from build123d import *

# Parameters (mm, degrees)
SKETCH1_W             = 24.5
SKETCH1_H             = 18.25
BOSS_EXTRUDE1_DEPTH   = 3
CHAMFER1_SIZE         = 0.75
CHAMFER2_SIZE         = 1.5
CHAMFER2_SIZE2        = 5.598076211
CHAMFER2_PART_2_SIZE  = 1.5
CHAMFER2_PART_2_SIZE2 = 5.598076211
CHAMFER2_PART_3_SIZE  = 1.5
CHAMFER2_PART_3_SIZE2 = 5.598076211
CHAMFER2_PART_4_SIZE  = 1.5
CHAMFER2_PART_4_SIZE2 = 5.598076211
SKETCH4_W             = 3
SKETCH4_H             = 0.5
BOSS_EXTRUDE2_DEPTH   = 2.5
FILLET2_R             = 1
FILLET2_OF_MIRROR2_R  = 1
SKETCH5_R             = 0.75
BOSS_EXTRUDE3_DEPTH   = 0.5
CUT_EXTRUDE2_REACH    = 23.288
SKETCH6_R             = 0.5


with BuildPart() as part:
    # Sketch1 → Boss-Extrude1 (new body)
    with BuildSketch(Plane(origin=(0, 0, 0), x_dir=(1, 0, 0), z_dir=(0, 1, 0))):
        Rectangle(SKETCH1_W, SKETCH1_H)
    extrude(amount=BOSS_EXTRUDE1_DEPTH)

    # Chamfer1
    chamfer1_edges = [part.edges().sort_by_distance(p)[0] for p in [
        (12.25, 1.5, 9.125),
        (-12.25, 1.5, 9.125),
        (-12.25, 1.5, -9.125),
        (12.25, 1.5, -9.125),
    ]]
    chamfer(chamfer1_edges, length=CHAMFER1_SIZE)

    # Chamfer2
    chamfer2_edges = [part.edges().sort_by_distance(p)[0] for p in [
        (12.25, 3, 0),
    ]]
    chamfer2_side = [part.faces().sort_by_distance(p)[0] for p in [
        (12.25, 1.5, 0),
    ]]
    chamfer(chamfer2_edges, length=CHAMFER2_SIZE, length2=CHAMFER2_SIZE2, reference=chamfer2_side[0])

    # Chamfer2 part 2
    chamfer2_part_2_edges = [part.edges().sort_by_distance(p)[0] for p in [
        (0, 3, 9.125),
    ]]
    chamfer2_part_2_side = [part.faces().sort_by_distance(p)[0] for p in [
        (0, 1.5, 9.125),
    ]]
    chamfer(chamfer2_part_2_edges, length=CHAMFER2_PART_2_SIZE, length2=CHAMFER2_PART_2_SIZE2, reference=chamfer2_part_2_side[0])

    # Chamfer2 part 3
    chamfer2_part_3_edges = [part.edges().sort_by_distance(p)[0] for p in [
        (-12.25, 3, 0),
    ]]
    chamfer2_part_3_side = [part.faces().sort_by_distance(p)[0] for p in [
        (-12.25, 1.5, 0),
    ]]
    chamfer(chamfer2_part_3_edges, length=CHAMFER2_PART_3_SIZE, length2=CHAMFER2_PART_3_SIZE2, reference=chamfer2_part_3_side[0])

    # Chamfer2 part 4
    chamfer2_part_4_edges = [part.edges().sort_by_distance(p)[0] for p in [
        (0, 3, -9.125),
    ]]
    chamfer2_part_4_side = [part.faces().sort_by_distance(p)[0] for p in [
        (0, 1.5, -9.125),
    ]]
    chamfer(chamfer2_part_4_edges, length=CHAMFER2_PART_4_SIZE, length2=CHAMFER2_PART_4_SIZE2, reference=chamfer2_part_4_side[0])

    # Sketch4 → Boss-Extrude2 (add)
    with BuildSketch(Plane.XZ):
        with Locations((0, 7.775)):
            Rectangle(SKETCH4_W, SKETCH4_H)
    boss_extrude2 = extrude(amount=BOSS_EXTRUDE2_DEPTH)

    # Fillet2
    fillet2_edges = [part.edges().sort_by_distance(p)[0] for p in [
        (-1.5, -2.5, 7.775),
        (1.5, -2.5, 7.775),
    ]]
    fillet(fillet2_edges, radius=FILLET2_R)

    # Mirror2: Boss-Extrude2 across plane
    add(boss_extrude2.mirror(Plane.XY))

    # Fillet2 of Mirror2
    fillet2_of_mirror2_edges = [part.edges().sort_by_distance(p)[0] for p in [
        (-1.5, -2.5, -7.775),
        (1.5, -2.5, -7.775),
    ]]
    fillet(fillet2_of_mirror2_edges, radius=FILLET2_OF_MIRROR2_R)

    # Sketch5 → Boss-Extrude3 (add)
    with BuildSketch(Plane(origin=(0, 0, -8.025), x_dir=(-1, 0, 0), z_dir=(0, 0, -1))):
        with Locations((0, -1.5)):
            Circle(SKETCH5_R)
    extrude(amount=BOSS_EXTRUDE3_DEPTH)

    # Sketch6 → Cut-Extrude2 (cut, up to next)
    with BuildSketch(Plane.XY.offset(8.025), mode=Mode.PRIVATE) as cut_extrude2_sk1:
        with Locations((0, -1.5)):
            Circle(SKETCH6_R)
    cut_extrude2_tool1 = extrude(cut_extrude2_sk1.sketch, amount=-CUT_EXTRUDE2_REACH, mode=Mode.PRIVATE) & part.part
    add(cut_extrude2_tool1.solids().sort_by_distance((0, -1.5, 8.025))[0], mode=Mode.SUBTRACT)


solid = part.part
Can you work these out from the model? Positions are in its coordinate system, mm. A direction names the side the tool comes from. Round coordinates to 2 decimals unless told otherwise and drop trailing zeros. Loops run counter-clockwise (first coordinate to the right, second up) from the corner with the lowest first, then second, coordinate; pieces in that order, holes last. Notation, with made-up numbers: (0.5, -18) - (39.5, -18) arc R20 cw to (39.5, 9) - close; hole circle Ø4 at (-37.75, 7). An arc over 180 degrees is marked (long way). Use CSV: the item, a comma, the result in double quotes. Start each with the question number.
1) We'd pull the mould along Y, two halves only. Please class faces 6 (the cylindrical face through (-1.215, -2.199, 7.778)), 7 (the flat face through (12.25, 1, 0)), 8 (the cylindrical face through (0.098, -0.756, -8.272)): released by +Y, released by -Y, zero draft, split by the parting line, or undercut.
2) If we section it at C-C on z = -4: Write out the boundary of the cut face in (x, y) (3 decimals).
3) Please list where these lines run through material, in increasing order: probe 1 along Z at (x, y) = (1, -0.05) (3 decimals); probe 2 along Y at (x, z) = (-4.5, -1); probe 3 along Y at (x, z) = (-10.5, -0.25). Write a range as [from, to].
4) If we section it at A-A on x = 0: Write out the boundary of the cut face in (y, z) (3 decimals).
5) If we section it at B-B on x = -4.75: Write out the boundary of the cut face in (y, z) (3 decimals), plus the area to 3 significant figures.
6) For faces 1 (the flat face through (10.034, 2.094, 0.123)), 2 (the flat face through (-0.35, -0.95, 8.025)), 3 (the flat face through (0, -1, -7.525)), 4 (the cylindrical face through (1.215, -2.199, 7.778)), 5 (the flat face through (1, -1, -8.025)), which set-ups out of +Z, -Z, +X, -X, +Y, -Y let a thin tool reach every point of the face, with its end or its side?
7) For pin 1 Ø2 at (x, z) = (-2.5, -5) entering from -Y; pin 2 Ø1.2 at (x, y) = (0.5, -1) entering from -Z (3 decimals), each with a flat end and sliding along its axis, tell me the tip position at first contact or that it passes through.
Geometry results:
1,face 6,"released by -Y"
1,face 7,"zero draft"
1,face 8,"undercut"
2,outline,"(-12.25, 0) - (12.25, 0) - (12.25, 1.5) - (7.125, 2.873) - (-7.125, 2.873) - (-12.25, 1.5) - close"
3,probe 1,"z = [-8.025, -7.525], [7.525, 8.025]"
3,probe 2,"y = [0, 3]"
3,probe 3,"y = [0, 1.97]"
4,outline,"(-2.5, -8.025) - (-2.25, -8.025) - (-2.25, -8.525) - (-0.75, -8.525) - (-0.75, -8.025) - (0, -8.025) - (0, -9.125) - (1.5, -9.125) - (3, -3.527) - (3, 3.527) - (1.5, 9.125) - (0, 9.125) - (0, 8.025) - (-1, 8.025) - (-1, 7.525) - (0, 7.525) - (0, -7.525) - (-2.5, -7.525) - close; (-2.5, 7.525) - (-2, 7.525) - (-2, 8.025) - (-2.5, 8.025) - close"
5,outline,"(0, -9.125) - (1.5, -9.125) - (3, -3.527) - (3, 3.527) - (1.5, 9.125) - (0, 9.125) - close"
5,area,"46.4 mm2"
6,face 1,"+Z, -Z, +X, +Y"
6,face 2,"+Z, +X, -X, -Y"
6,face 3,"+X, -X, -Y"
6,face 4,"+Z, -Z, +X, -Y"
6,face 5,"-Z"
7,pin 1,"stops at y = 0"
7,pin 2,"stops at z = -8.525"
